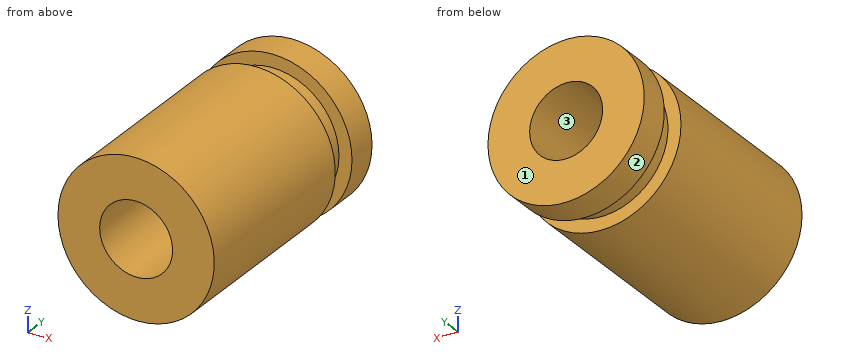
Autodesk Inventor part; units mm, degrees
ref_plane "YZ Plane" through (0, 0, 0) normal (1, 0, 0) x (0, 1, 0)
ref_plane "XZ Plane" through (0, 0, 0) normal (0, 1, 0) x (-1, 0, 0)
ref_plane "XY Plane" through (0, 0, 0) normal (0, 0, 1) x (1, 0, 0)
sketch "Esboço1" plane through (0, 0, 0) normal (0, 1, 0) x (-1, 0, 0)
  circle A0 centre (0, 0) radius 15
  dimension "d0" = 30
extrude "Extrusão1" add sketch "Esboço1" along normal blind 36.24
sketch "Esboço2" plane through (0, 36.24, 0) normal (0, 1, 0) x (1, 0, 0)
  circle A0 centre (0, 0) radius 12.5
  dimension "d3" = 25
extrude "Extrusão2" add sketch "Esboço2" along normal blind 5
sketch "Esboço3" plane through (0, 41.24, 0) normal (0, 1, 0) x (1, 0, 0)
  circle A0 centre (0, 0) radius 15
extrude "Extrusão3" add sketch "Esboço3" along normal blind 6
sketch "Sketch5" plane through (0, 47.24, 0) normal (0, 1, 0) x (1, 0, 0)
  circle A0 centre (0, 0) radius 15
hole "Hole2" at (0, 47.24, 0) direction (0, -1, 0) diameter 14 end through all
thread "Thread1"
equation "\"d20\" = Espessura"
equation "\"Raio_vergadura\" = Espessura"
equation "\"Largura_alívio_de_vergadura\" = Espessura"
equation "\"Profundidade_alívio_de_vergadura\" = 0.5 * Espessura"
equation "\"Tamanho_alívio_de_dobra\" = 4 * Espessura"
equation "\"Remanescente_mínimo\" = 2 * Espessura"
equation "\"Raiodetransição\" = Raio_vergadura"
equation "\"Tamanho_de_raio_de_Jacobi\" = Raio_vergadura"
equation "\"TamanhoFolga\" = Espessura"
properties part number "Guia do eixo roscado" material "Aço"
For this review, take the finished solid that the model builds, in its own axes (mm). Face numbers are marked on the shaded views. Round coordinates to 2 decimals unless told otherwise and drop trailing zeros. Order: outer loops, then holes, each group sorted by start corner. A loop starts at its lowest first (then second) coordinate and runs counter-clockwise, first axis right, second up. Notation, with made-up numbers: M 32,62.5 L 62,62.5 A22 ccw 62,74.5 Z; hole C 82.25,-18.5 d9. An arc over 180 degrees is marked long. Write each question's results on one line, items separated by ' | '. Start each with the question number.
1. To check wall thickness, follow L1, parallel to X at y = 37, z = 0; L2, parallel to Y at x = -9.5, z = -8.25; L3, parallel to Z at x = 0, y = 26. State the ranges of each line that lie inside material, in increasing order. Write a range as [from, to].
2. Draft analysis for pull direction X (two halves, no side actions). For the marked faces 1, 2 and 3, state which applies: pulls with the +X half, pulls with the -X half, needs draft (parallel to the pull), parting line crosses it, or undercut.
3. Add section A-A (x = 0). State the section outline as (y, z) points.
4. Add section C-C (y = 38). State the section outline as (x, z) points, then the cut area to 3 significant figures.
5. Add section D-D (z = -9.75). State the section outline as (x, y) points, then the cut area to 3 significant figures.
6. Clearance check with flat-ended pins moving along their axes: pin 1 Ø4 at (x, y) = (-8, 8) entering from +Z; pin 2 Ø6 at (y, z) = (8.5, 7.5) entering from -X; pin 3 Ø2 at (y, z) = (39, 7.5) entering from -X. State where each tip first meets the part, or that it passes through.
7. Add section B-B (z = 0). State the section outline as (x, y) points, then the cut area to 3 significant figures.
Output values:
1) L1: [-12.5, -7], [7, 12.5] | L2: [0, 36.24], [41.24, 47.24] | L3: [-15, -7], [7, 15]
2) face 1: needs draft | face 2: parting line crosses it | face 3: undercut
3) outline: M 0,-15 L 36.24,-15 L 36.24,-12.5 L 41.24,-12.5 L 41.24,-15 L 47.24,-15 L 47.24,-7 L 0,-7 Z; M 0,7 L 47.24,7 L 47.24,15 L 41.24,15 L 41.24,12.5 L 36.24,12.5 L 36.24,15 L 0,15 Z
4) outline: C 0,0 d25; hole C 0,0 d14 | area: 337 mm^2
5) outline: M -11.4,0 L 11.4,0 L 11.4,36.24 L 7.82,36.24 L 7.82,41.24 L 11.4,41.24 L 11.4,47.24 L -11.4,47.24 L -11.4,41.24 L -7.82,41.24 L -7.82,36.24 L -11.4,36.24 Z | area: 1,040 mm^2
6) pin 1: z = 13.75 | pin 2: x = -14.31 | pin 3: x = -10.68
7) outline: M -15,0 L -7,0 L -7,47.24 L -15,47.24 L -15,41.24 L -12.5,41.24 L -12.5,36.24 L -15,36.24 Z; M 7,0 L 15,0 L 15,36.24 L 12.5,36.24 L 12.5,41.24 L 15,41.24 L 15,47.24 L 7,47.24 Z | area: 731 mm^2
